Source: CAD feature listing. Evaluate the final solid. Frame: model axes, mm. Round coordinates to 2 decimals unless told otherwise and drop trailing zeros. Write each loop counter-clockwise with the first axis right and the second up, starting at its lowest first coordinate (ties: lowest second). Pieces come first, ordered by that corner, then holes. Notation, with made-up numbers: (49.5, -9) -> (54.5, -9) arc R20 ccw to (54.5, -2) -> close; hole circle Ø2 at (-18.5, -32.75). An arc over 180 degrees is marked (long way). Put each result on its own line as item: value.
```python
from build123d import *

# Parameters (mm, degrees)
SKETCH1_R           = 2
SKETCH1_W           = 40
SKETCH1_H           = 60
SKETCH1_R_2         = 1.5
SKETCH1_R_3         = 2.5
BOSS_EXTRUDE1_DEPTH = 5
FILLET1_R           = 6
SKETCH2_R           = 1.5
CUT_EXTRUDE1_DEPTH  = 296.88849251


with BuildPart() as part:
    # Sketch1 → Boss-Extrude1 (new body)
    with BuildSketch(Plane(origin=(0, 0, 0), x_dir=(1, 0, 0), z_dir=(0, 1, 0))):
        Polygon((-150, 210), (-150, -210), (150, -210), (150, 210), (150, 255), (-150, 255), align=None)
        with Locations(Location((-140, -200, 0), (0, 0, 270))):
            Circle(SKETCH1_R, mode=Mode.SUBTRACT)
        with Locations((-110, -160)):
            Rectangle(SKETCH1_W, SKETCH1_H, mode=Mode.SUBTRACT)
        with Locations(Location((-140, -140, 0), (0, 0, 270))):
            Circle(SKETCH1_R, mode=Mode.SUBTRACT)
        with Locations(Location((-140, -40, 0), (0, 0, 270))):
            Circle(SKETCH1_R, mode=Mode.SUBTRACT)
        with Locations(Location((0, -200, 0), (0, 0, 270))):
            Circle(SKETCH1_R, mode=Mode.SUBTRACT)
        with Locations((110, -160)):
            Rectangle(SKETCH1_W, SKETCH1_H, mode=Mode.SUBTRACT)
        with Locations(Location((140, -200, 0), (0, 0, 270))):
            Circle(SKETCH1_R, mode=Mode.SUBTRACT)
        with Locations(Location((140, -140, 0), (0, 0, 270))):
            Circle(SKETCH1_R, mode=Mode.SUBTRACT)
        with Locations(Location((140, -40, 0), (0, 0, 270))):
            Circle(SKETCH1_R, mode=Mode.SUBTRACT)
        with Locations(Location((-140, 60, 0), (0, 0, 270))):
            Circle(SKETCH1_R, mode=Mode.SUBTRACT)
        with Locations(Location((-144, 125.375, 0), (0, 0, 270))):
            Circle(SKETCH1_R_2, mode=Mode.SUBTRACT)
        with Locations(Location((-114, 125.375, 0), (0, 0, 270))):
            Circle(SKETCH1_R_2, mode=Mode.SUBTRACT)
        with Locations(Location((-84, 125.375, 0), (0, 0, 270))):
            Circle(SKETCH1_R_2, mode=Mode.SUBTRACT)
        with Locations(Location((-144, 182.625, 0), (0, 0, 270))):
            Circle(SKETCH1_R_2, mode=Mode.SUBTRACT)
        with Locations(Location((-114, 182.625, 0), (0, 0, 270))):
            Circle(SKETCH1_R_2, mode=Mode.SUBTRACT)
        with Locations(Location((-84, 182.625, 0), (0, 0, 270))):
            Circle(SKETCH1_R_2, mode=Mode.SUBTRACT)
        with Locations(Location((-140, 200, 0), (0, 0, 270))):
            Circle(SKETCH1_R, mode=Mode.SUBTRACT)
        with Locations(Location((-140, 248, 0), (0, 0, 270))):
            Circle(SKETCH1_R_3, mode=Mode.SUBTRACT)
        with Locations(Location((140, 60, 0), (0, 0, 270))):
            Circle(SKETCH1_R, mode=Mode.SUBTRACT)
        with Locations(Location((84, 125.375, 0), (0, 0, 270))):
            Circle(SKETCH1_R_2, mode=Mode.SUBTRACT)
        with Locations(Location((114, 125.375, 0), (0, 0, 270))):
            Circle(SKETCH1_R_2, mode=Mode.SUBTRACT)
        with Locations(Location((144, 125.375, 0), (0, 0, 270))):
            Circle(SKETCH1_R_2, mode=Mode.SUBTRACT)
        with Locations(Location((0, 200, 0), (0, 0, 270))):
            Circle(SKETCH1_R, mode=Mode.SUBTRACT)
        with Locations(Location((84, 182.625, 0), (0, 0, 270))):
            Circle(SKETCH1_R_2, mode=Mode.SUBTRACT)
        with Locations(Location((114, 182.625, 0), (0, 0, 270))):
            Circle(SKETCH1_R_2, mode=Mode.SUBTRACT)
        with Locations(Location((144, 182.625, 0), (0, 0, 270))):
            Circle(SKETCH1_R_2, mode=Mode.SUBTRACT)
        with Locations(Location((140, 200, 0), (0, 0, 270))):
            Circle(SKETCH1_R, mode=Mode.SUBTRACT)
        with Locations(Location((140, 248, 0), (0, 0, 270))):
            Circle(SKETCH1_R_3, mode=Mode.SUBTRACT)
    extrude(amount=BOSS_EXTRUDE1_DEPTH)

    # Fillet1
    fillet1_edges = [part.edges().sort_by_distance(p)[0] for p in [
        (130, 2.5, 190),
        (130, 2.5, 130),
        (90, 2.5, 130),
        (90, 2.5, 190),
        (-90, 2.5, 130),
        (-130, 2.5, 130),
        (-130, 2.5, 190),
        (-90, 2.5, 190),
        (-150, 2.5, -255),
        (150, 2.5, -255),
    ]]
    fillet(fillet1_edges, radius=FILLET1_R)

    # Sketch2 → Cut-Extrude1 (cut, through all)
    with BuildSketch(Plane(origin=(0, 5, 0), x_dir=(1, 0, 0), z_dir=(0, 1, 0))):
        with Locations(Location((-18, -144, 0), (0, 0, 270))):
            Circle(SKETCH2_R)
        with Locations(Location((18, -144, 0), (0, 0, 270))):
            Circle(SKETCH2_R)
        with Locations(Location((18, -84, 0), (0, 0, 270))):
            Circle(SKETCH2_R)
        with Locations(Location((-18, -84, 0), (0, 0, 270))):
            Circle(SKETCH2_R)
        with Locations(Location((-120, -69, 0), (0, 0, 270))):
            Circle(SKETCH2_R)
        with Locations(Location((120, -69, 0), (0, 0, 270))):
            Circle(SKETCH2_R)
        with Locations(Location((120, 111, 0), (0, 0, 270))):
            Circle(SKETCH2_R)
        with Locations(Location((-120, 111, 0), (0, 0, 270))):
            Circle(SKETCH2_R)
        with Locations(Location((0, 22.5, 0), (0, 0, 270))):
            Circle(SKETCH2_R)
    extrude(amount=-CUT_EXTRUDE1_DEPTH, mode=Mode.SUBTRACT)


solid = part.part
```
Q1. Material intervals for line 1 (X direction, y = 3.9, z = 158.5); line 2 (X direction, y = 1.5, z = -248); line 3 (Z direction, x = -84, y = 3.1) (3 decimals), sorted ascending. Write a range as [from, to].
Ans:
line 1: x = [-150, -130], [-90, 90], [130, 150]
line 2: x = [-150, -142.5], [-137.5, 137.5], [142.5, 150]
line 3: z = [-255, -184.125], [-181.125, -126.875], [-123.875, 210]
Q2. Cut plane A-A on z = 170. Output: boundary loops of the cut face in (x, y), and give its area (3 significant figures).
Ans:
outline: (-150, 0) -> (-130, 0) -> (-130, 5) -> (-150, 5) -> close; (-90, 0) -> (90, 0) -> (90, 5) -> (-90, 5) -> close; (130, 0) -> (150, 0) -> (150, 5) -> (130, 5) -> close
area: 1,100 mm^2
Q3. Cut plane B-B on y = 0.9. Give the number of separate pieces and of enclosed holes in the cut face, and give its area (3 significant figures).
Ans:
separate pieces: 1
enclosed holes: 37
area: 134,000 mm^2
Q4. Pin query (flat end, axial travel): pin 1 (4 mm diameter, centred on x = 114, z = -125.375, fed in from -Y); pin 2 (2.5 mm diameter, centred on x = 140, z = 140, fed in from -Y). Return the tip coordinate at first contact, or that it passes through.
Ans:
pin 1: stops at y = 0
pin 2: passes through
